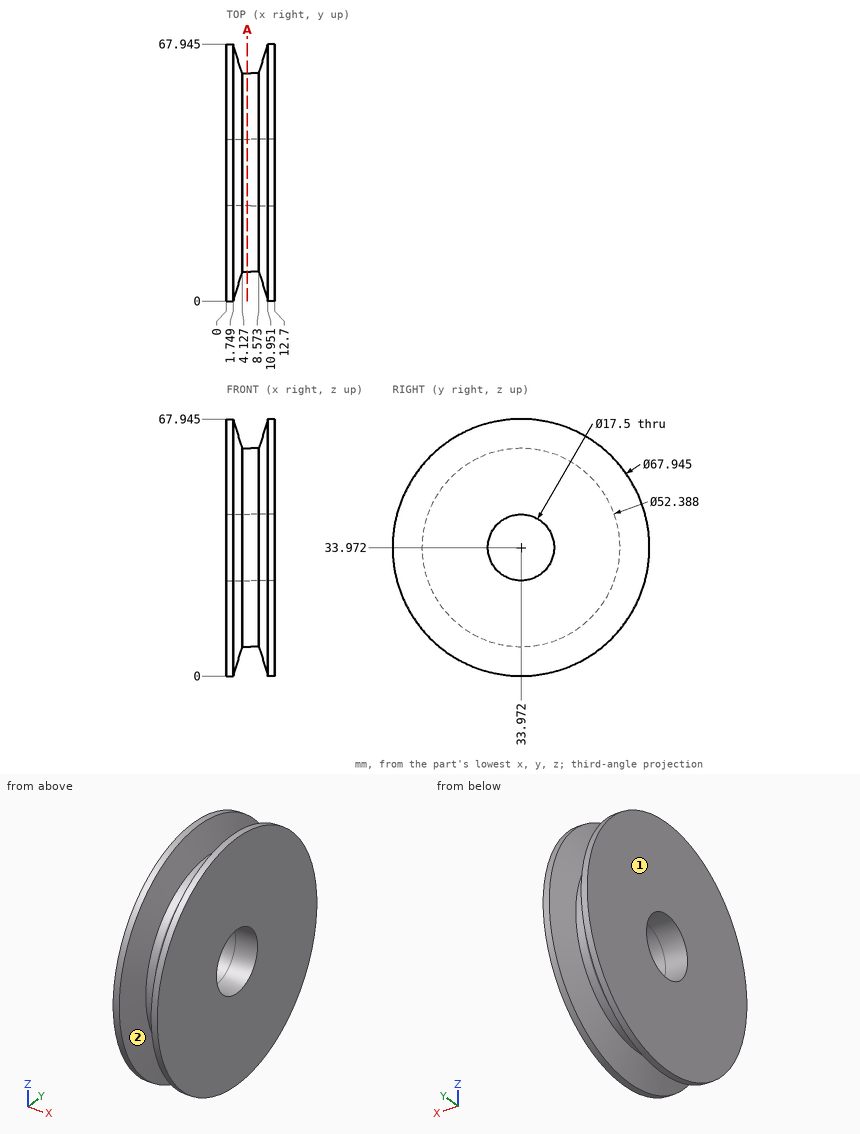
Part print with two shaded views. Sizes in mm from the minimum x, y, z corner. A direction names the side the tool comes from. Round coordinates to 2 decimals unless told otherwise and drop trailing zeros. Order: outer loops, then holes, each group sorted by start corner. A loop starts at its lowest first (then second) coordinate and runs counter-clockwise, first axis right, second up.
(1) 3-axis set-ups, long thin cutter, end or side, ignore diameter. For the marked faces 1 and 2: which of +Z, -Z, +X, -X, +Y, -Y reach the whole face in a straight line?
(2) Drill centre lines: line 1 (Y direction, x = 5.25, z = 34.5) (1 decimal); line 2 (X direction, y = 7.5, z = 51.5); line 3 (X direction, y = 10, z = 12). Where is each one in solid material? Low to high.
(3) Band-saw the part on A-A (x = 5.5). List the corners of the cut face in (y, z).
(4) Pin check, flat tips, straight feed: pin 1 (1.5 mm diameter, centred on x = 7, y = 11, fed in from -Z) (1 decimal); pin 2 (6 mm diameter, centred on x = 3.5, y = 11.5, fed in from +Z); pin 3 (2 mm diameter, centred on x = 2.5, y = 41, fed in from +Z). Stop position of each tip, or through.
Verdict:
1. face 1: +Z, -Z, -X, +Y, -Y
1. face 2: none
2. line 1: y = 7.8 to 25.2, 42.7 to 60.2
2. line 2: x = 0 to 2.43, 10.27 to 12.7
2. line 3: x = 0 to 2.19, 10.51 to 12.7
3. outline: circle Ø52.39 at (33.97, 33.97); hole circle Ø17.5 at (33.97, 33.97)
4. pin 1: stops at z = 20.1
4. pin 2: stops at z = 61.41
4. pin 3: stops at z = 67.34
